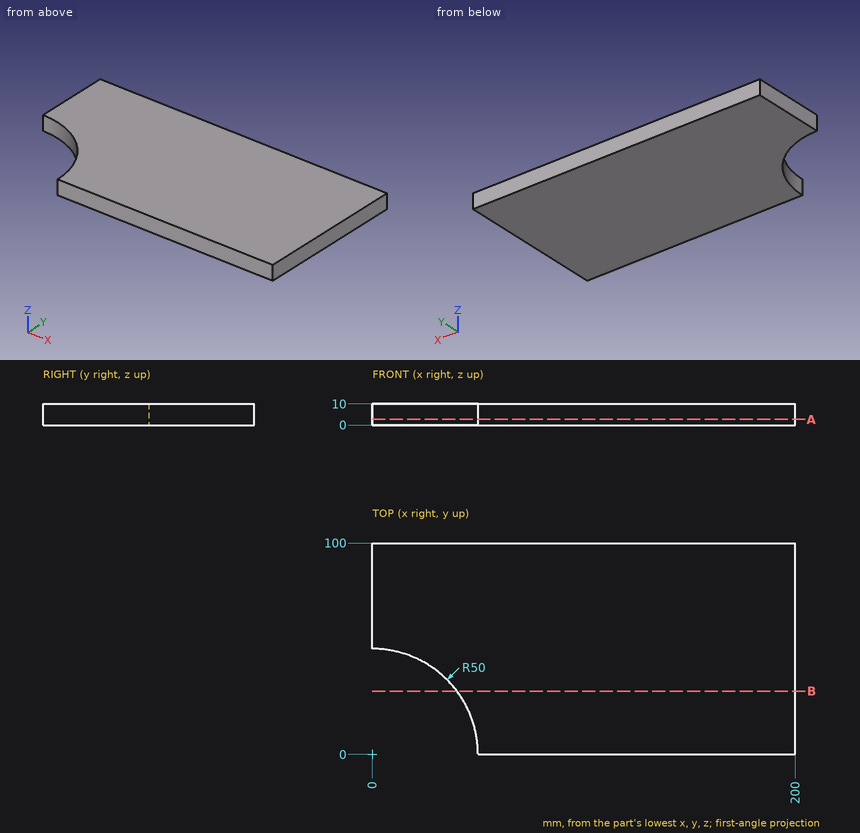
Here's the drawing with two shaded views (mm, measured from the low corner). I have some questions. Give positions to 0.01 mm unless a question says otherwise; leave off trailing zeros. Write each loop counter-clockwise with the first axis right and the second up, starting at its lowest first coordinate (ties: lowest second). Pieces come first, ordered by that corner, then holes. Notation, with made-up numbers: (77, -7.5) - (98, -7.5) arc R22 cw to (98, 9.5) - close; hole circle Ø11 at (10.25, -12.75). An arc over 180 degrees is marked (long way). One line per item, written item: value. Start each with the question number.
Item 1: I'm going to push a flat-ended pin straight in: pin 1 (1 mm diameter, centred on y = 35, z = 9, fed in from -X). Where does the tip first touch, or does it pass through?
Item 2: Please list where these lines run through material, in increasing order: line 1 (X direction, y = 9.5, z = 6.5); line 2 (Y direction, x = 10.5, z = 1.5); line 3 (X direction, y = 44, z = 9.75). Write a range as from..to.
Item 3: Imagine slicing it at B-B, the plane y = 30. List the corners of the cut face in (x, z) for me.
Item 4: Imagine slicing it at A-A, the plane z = 2.75. List the corners of the cut face in (x, y) for me, and give its area (3 significant figures).
Geometry says:
1. pin 1: x = 35.21
2. line 1: 49.09..200
2. line 2: 48.89..100
2. line 3: 23.75..200
3. outline: (40, 0) - (200, 0) - (200, 10) - (40, 10) - close
4. outline: (0, 50) arc R50 cw to (50, 0) - (200, 0) - (200, 100) - (0, 100) - close
4. area: 18,000 mm^2
